Geometry check sheet. Reference: the model listing, model coordinates, mm. A direction names the side the tool comes from. Round coordinates to 2 decimals unless told otherwise and drop trailing zeros. Loops run counter-clockwise (first coordinate to the right, second up) from the corner with the lowest first, then second, coordinate; pieces in that order, holes last. Notation, with made-up numbers: (17.5, 30) -> (52.5, 30) arc R6 cw to (52.5, 39) -> close; hole circle Ø5 at (-34.75, -7.5). An arc over 180 degrees is marked (long way). Use one line per item in the form item = value.
from build123d import *

# Parameters (mm, degrees)
SKETCH1_R               = 2.285
BOSS_EXTRUDE1_DEPTH     = 8
SKETCH2_R               = 15
BOSS_EXTRUDE2_DEPTH     = 15
CUT_EXTRUDE1_DEPTH      = 18
CUT_EXTRUDE1_DEPTH_BACK = 2
SKETCH3_R               = 3.5
CUT_EXTRUDE2_START      = 10.222
SKETCH4_R               = 7.7375
CUT_EXTRUDE2_DEPTH      = 6
FILLET1_R               = 8
FILLET2_R               = 2
CHAMFER1_SIZE           = 2


with BuildPart() as part:
    # Sketch1 → Boss-Extrude1 (new body)
    with BuildSketch(Plane.XY):
        Polygon((-135.206606908, -69.673474959), (-135.206606908, 30.326525041), (31.793393092, 80.326525041), (98.793393092, 30.326525041), (98.793393092, -69.673474959), align=None)
        with Locations((-125.206606908, 5.326525041)):
            Circle(SKETCH1_R, mode=Mode.SUBTRACT)
        with Locations((-95.206606908, -59.673474959)):
            Circle(SKETCH1_R, mode=Mode.SUBTRACT)
        with Locations((59.312548963, 47.312193908)):
            Circle(SKETCH1_R, mode=Mode.SUBTRACT)
        with Locations((-48.838391267, 45.7466848)):
            Circle(SKETCH1_R, mode=Mode.SUBTRACT)
        with Locations(Location((58.793393092, -59.673474959, 0), (0, 0, 180))):
            Circle(SKETCH1_R, mode=Mode.SUBTRACT)
        with Locations(Location((-125.206606908, -54.673474959, 0), (0, 0, 180))):
            Circle(SKETCH1_R, mode=Mode.SUBTRACT)
        with Locations((88.793393092, -54.673474959)):
            Circle(SKETCH1_R, mode=Mode.SUBTRACT)
        with Locations((88.793393092, -9.673474959)):
            Circle(SKETCH1_R, mode=Mode.SUBTRACT)
    extrude(amount=BOSS_EXTRUDE1_DEPTH)

    # Sketch2 → Boss-Extrude2 (add)
    with BuildSketch(Plane.XY):
        with Locations(Location((71.793393092, 5.326525041, 0), (0, 0, 180))):
            Circle(SKETCH2_R)
    extrude(amount=BOSS_EXTRUDE2_DEPTH)

    # Sketch3 → Cut-Extrude1 (cut, two sides: drawn at the far end of the back side and taken through both)
    with BuildSketch(Plane.XY.offset(-CUT_EXTRUDE1_DEPTH_BACK)):
        with Locations((71.793393092, 5.326525041)):
            Circle(SKETCH3_R)
        with BuildLine():
            Line((44.668393092, -69.673474959), (44.668393092, -64.543474959))
            Line((44.668393092, -64.543474959), (23.668393092, -64.543474959))
            Line((23.668393092, -64.543474959), (23.668393092, -24.673474959))
            ThreePointArc((23.668393092, -24.673474959), (-18.206606908, 17.201525041), (-60.081606908, -24.673474959))
            Line((-60.081606908, -24.673474959), (-60.081606908, -64.543474959))
            Line((-60.081606908, -64.543474959), (-81.081606908, -64.543474959))
            Line((-81.081606908, -64.543474959), (-81.081606908, -69.673474959))
            Line((-81.081606908, -69.673474959), (-81.081606908, -72.333497989))
            Line((-81.081606908, -72.333497989), (44.668393092, -72.333497989))
            Line((44.668393092, -72.333497989), (44.668393092, -69.673474959))
        make_face()
    extrude(amount=CUT_EXTRUDE1_DEPTH + CUT_EXTRUDE1_DEPTH_BACK, mode=Mode.SUBTRACT)

    # Sketch4 → Cut-Extrude2 (cut)
    with BuildSketch(Plane.XY.offset(CUT_EXTRUDE2_START)):
        with Locations((71.793393092, 5.326525041)):
            Circle(SKETCH4_R)
    extrude(amount=CUT_EXTRUDE2_DEPTH, mode=Mode.SUBTRACT)

    # Fillet1
    fillet1_edges = [part.edges().sort_by_distance(p)[0] for p in [
        (23.668393092, -64.543474959, 4),
        (-60.081606908, -64.543474959, 4),
    ]]
    fillet(fillet1_edges, radius=FILLET1_R)

    # Fillet2
    fillet2_edges = [part.edges().sort_by_distance(p)[0] for p in [
        (-81.081606908, -64.543474959, 4),
        (44.668393092, -64.543474959, 4),
    ]]
    fillet(fillet2_edges, radius=FILLET2_R)

    # Chamfer1
    chamfer1_edges = [part.edges().sort_by_distance(p)[0] for p in [
        (86.793393092, 5.326525041, 8),
    ]]
    chamfer(chamfer1_edges, length=CHAMFER1_SIZE)


solid = part.part
1. Section check D-D (y = 34.5). Record the boundary of the cut face in (x, z).
Return value:
outline = (-121.27, 0) -> (93.2, 0) -> (93.2, 8) -> (-121.27, 8) -> close
2. Tool access check on faces 1 (the cylindrical face through (-46.66, 46.43, 3.94)), 2 (the cylindrical face through (57.937, 11.072, 12.465)), 3 (the cylindrical face through (-62.363, -62.138, 4.056)). Record the directions out of +Z, -Z, +X, -X, +Y, -Y that give a thin tool (end or side, any length) a straight path to the whole face; none if there is none.
Return value:
face_1 = +Z, -Z
face_2 = +Z
face_3 = +Z, -Z, -Y
3. Mould release check, pull along Y, two halves, no side actions. Record for faces 4 (the flat face through (72, -69.673, 4)), 5 (the flat face through (-135.207, -20, 4)), 6 (the cylindrical face through (58.82, 45.08, 3.94)): released by +Y, released by -Y, zero draft, split by the parting line, or undercut.
Return value:
face_4 = released by -Y
face_5 = zero draft
face_6 = undercut
4. Section check B-B (z = 2.25). Count the separate pieces of the cut face and the enclosed holes in it, then the cut area to 3 significant figures.
Return value:
separate_pieces = 1
enclosed_holes = 9
area = 22,300 mm2
5. Material ranges on line 1 along X through (y, z) = (-23.5, 2.5); line 2 along Z through (x, y) = (77, -26.5); line 3 along X through (y, z) = (-61.5, 4), recorded low to high.
Return value:
line_1 = -135.21 to -60.07, 23.65 to 98.79
line_2 = 0 to 8
line_3 = -135.21 to -96.58, -93.83 to -61.8, 25.39 to 57.42, 60.17 to 98.79
6. Section check A-A (y = -47). Record the boundary of the cut face in (x, z).
Return value:
outline = (-135.21, 0) -> (-60.08, 0) -> (-60.08, 8) -> (-135.21, 8) -> close; (23.67, 0) -> (98.79, 0) -> (98.79, 8) -> (23.67, 8) -> close
7. Section check C-C (x = 15). Record the boundary of the cut face in (y, z).
Return value:
outline = (0.84, 0) -> (75.3, 0) -> (75.3, 8) -> (0.84, 8) -> close
8. Gauge pin test, flat ends, axial feed: pin 1 (6.5 mm diameter, centred on x = 39.5, z = 5.5, fed in from -Y); pin 2 (7.5 mm diameter, centred on x = 88.79, y = -9.67, fed in from +Z); pin 3 (2 mm diameter, centred on y = 0.5, z = 13, fed in from -X). Record the tip position at first contact, or that the pin passes through.
Return value:
pin_1 = -64.55
pin_2 = 8
pin_3 = 57.29
